from build123d import *

# Parameters (mm, degrees)
SKETCH1_W           = 230
SKETCH1_H           = 173
BOSS_EXTRUDE1_DEPTH = 6
SKETCH2_W           = 228
SKETCH2_H           = 171
CUT_EXTRUDE1_DEPTH  = 5
SKETCH3_W           = 10
SKETCH3_H           = 30
CUT_EXTRUDE2_DEPTH  = 145.025171411


with BuildPart() as part:
    # Sketch1 → Boss-Extrude1 (new body)
    with BuildSketch(Plane(origin=(0, 0, 0), x_dir=(1, 0, 0), z_dir=(0, 1, 0))):
        Rectangle(SKETCH1_W, SKETCH1_H)
    extrude(amount=BOSS_EXTRUDE1_DEPTH)

    # Sketch2 → Cut-Extrude1 (cut)
    with BuildSketch(Plane(origin=(0, 0, 0), x_dir=(1, 0, 0), z_dir=(0, 1, 0))):
        Rectangle(SKETCH2_W, SKETCH2_H)
    extrude(amount=CUT_EXTRUDE1_DEPTH, mode=Mode.SUBTRACT)

    # Sketch3 → Cut-Extrude2 (cut, through all)
    with BuildSketch(Plane(origin=(0, 6, 0), x_dir=(1, 0, 0), z_dir=(0, 1, 0))):
        with Locations((110, -61.5)):
            Rectangle(SKETCH3_W, SKETCH3_H)
        with Locations((-110, 61.5)):
            Rectangle(SKETCH3_W, SKETCH3_H)
    extrude(amount=-CUT_EXTRUDE2_DEPTH, mode=Mode.SUBTRACT)


solid = part.part
Input: part model. Units: mm. Frame: model coordinates. A direction names the side the tool comes from. Give positions to 0.01 mm unless a question says otherwise; leave off trailing zeros. Write each loop counter-clockwise with the first axis right and the second up, starting at its lowest first coordinate (ties: lowest second). Pieces come first, ordered by that corner, then holes. Notation, with made-up numbers: M 85,16 L 120,16 A13 cw 120,21 Z; hole C 16.5,5.5 d7. An arc over 180 degrees is marked long. Write item = value, one per line. Start each with the question number.
1) Draft query along Z for faces 1 (the flat face through (-2, 2, 85.5)), 2 (the flat face through (-115, 3, -81)), 3 (the flat face through (-2, 3, -86.5)), 4 (the flat face through (111.5, 5.5, 46.5)). Return one class per face: +Z half, -Z half, draft (parallel to the pull), parting line (faces both ways), or undercut.
2) Cut plane C-C on z = 32.5. Return the cut outline in (x, y).
3) Cut plane D-D on z = 51.5. Return the cut outline in (x, y).
4) Reachability of faces 5 (the flat face through (-2, 2, -85.5)), 6 (the flat face through (-111.5, 5.2, -76.5)), 7 (the flat face through (-2, 6, -1)), 8 (the flat face through (115, 3, 82)), 9 (the flat face through (111.5, 5.5, 76.5)) from +Z, -Z, +X, -X, +Y, -Y: full face, straight path, thin tool, end or side. Return the list, or none.
5) Material intervals for line 1 along Z through (x, y) = (-8.5, 1.45); line 2 along X through (y, z) = (0.9, 3.5); line 3 along Y through (x, z) = (103, -48.5), sorted ascending. Write a range as [from, to].
6) First-contact query: pin 1 Ø1 at (x, z) = (19, 42) entering from -Y; pin 2 Ø1.1 at (y, z) = (5.5, -67) entering from -X; pin 3 Ø0.5 at (y, z) = (5.5, 64.5) entering from +X. Flat tips, straight axial feed; report the tip coordinate or a pass-through.
7) Cut plane B-B on x = -26. Return the cut outline in (y, z), then the cut area to 3 significant figures.
8) Cut plane A-A on y = 2.5. Return the cut outline in (x, z), then the cut area to 3 significant figures.
Solved:
q1.face_1 = undercut
q1.face_2 = draft
q1.face_3 = -Z half
q1.face_4 = undercut
q2.outline = M -115,0 L -114,0 L -114,5 L 114,5 L 114,0 L 115,0 L 115,6 L -115,6 Z
q3.outline = M -115,0 L -114,0 L -114,5 L 105,5 L 105,6 L -115,6 Z
q4.face_5 = -Y
q4.face_6 = -X, +Y, -Y
q4.face_7 = +Z, -Z, +X, -X, +Y
q4.face_8 = +Z, -Z, +X, +Y, -Y
q4.face_9 = +X, +Y, -Y
q5.line_1 = [-86.5, -85.5], [85.5, 86.5]
q5.line_2 = [-115, -114], [114, 115]
q5.line_3 = [5, 6]
q6.pin_1 = 5
q6.pin_2 = -105
q6.pin_3 = 105
q7.outline = M 0,-86.5 L 6,-86.5 L 6,86.5 L 0,86.5 L 0,85.5 L 5,85.5 L 5,-85.5 L 0,-85.5 Z
q7.area = 183 mm2
q8.outline = M -115,-86.5 L 115,-86.5 L 115,46.5 L 114,46.5 L 114,-85.5 L -114,-85.5 L -114,-76.5 L -115,-76.5 Z; M -115,-46.5 L -114,-46.5 L -114,85.5 L 114,85.5 L 114,76.5 L 115,76.5 L 115,86.5 L -115,86.5 Z
q8.area = 742 mm2
